from build123d import *

# Parameters (mm, degrees)
SKETCH1_R           = 4.5
BOSS_EXTRUDE3_DEPTH = 40
SKETCH4_R           = 3.5
CUT_EXTRUDE3_DEPTH  = 0.5
SKETCH5_R           = 3
CUT_EXTRUDE4_DEPTH  = 5
SKETCH6_R           = 2
BOSS_EXTRUDE4_DEPTH = 1
SKETCH7_R           = 0.6
BOSS_EXTRUDE5_DEPTH = 3.5
CHAMFER1_SIZE       = 0.4
CHAMFER1_SIZE2      = 0.145588094
FILLET1_R           = 0.2
CHAMFER2_SIZE       = 40
CHAMFER2_SIZE_2     = 0.698202597
FILLET2_R           = 0.5


# Read off the part's stored shape, not the designer's step: Dome1
with BuildPart() as part:
    # Sketch1 → Boss-Extrude3 (new body)
    with BuildSketch(Plane(origin=(0, 0, 0), x_dir=(1, 0, 0), z_dir=(0, 1, 0))):
        with Locations(Location((0, 0, 0), (0, 0, 270))):
            Circle(SKETCH1_R)
    extrude(amount=BOSS_EXTRUDE3_DEPTH)

    # Sketch4 → Cut-Extrude3 (cut)
    with BuildSketch(Plane.XZ):
        with Locations(Location((0, 0, 0), (0, 0, 270))):
            Circle(SKETCH4_R)
    extrude(amount=-CUT_EXTRUDE3_DEPTH, mode=Mode.SUBTRACT)

    # Sketch5 → Cut-Extrude4 (cut)
    with BuildSketch(Plane.XZ.offset(-0.5)):
        with Locations(Location((0, 0, 0), (0, 0, 270))):
            Circle(SKETCH5_R)
    extrude(amount=-CUT_EXTRUDE4_DEPTH, mode=Mode.SUBTRACT)

    # Sketch6 → Boss-Extrude4 (add)
    with BuildSketch(Plane.XZ.offset(-5.5)):
        with Locations(Location((0, 0, 0), (0, 0, 270))):
            Circle(SKETCH6_R)
    extrude(amount=BOSS_EXTRUDE4_DEPTH)

    # Sketch7 → Boss-Extrude5 (add)
    with BuildSketch(Plane.XZ.offset(-4.5)):
        with Locations(Location((0, 0, 0), (0, 0, 270))):
            Circle(SKETCH7_R)
    extrude(amount=BOSS_EXTRUDE5_DEPTH)

    # Chamfer1
    chamfer1_edges = [part.edges().sort_by_distance(p)[0] for p in [
        (0, 1, 0.6),
    ]]
    chamfer1_side = [part.faces().sort_by_distance(p)[0] for p in [
        (0, 2.75, 0.6),
    ]]
    chamfer(chamfer1_edges, length=CHAMFER1_SIZE, length2=CHAMFER1_SIZE2, reference=chamfer1_side[0])

    # Fillet1
    fillet1_edges = [part.edges().sort_by_distance(p)[0] for p in [
        (0, 1, 0.454411906),
    ]]
    fillet(fillet1_edges, radius=FILLET1_R)

    # Chamfer2
    # the kernel refuses this chamfer: 40, 0.698202597 mm, written as the material it takes off along each edge
    with BuildSketch(Plane(origin=(0, 40, 0), x_dir=(0, 0, 1), z_dir=(-1, 0, 0))) as chamfer2_piece_1:
        Polygon((4.5, -CHAMFER2_SIZE), (4.5 - CHAMFER2_SIZE_2, 0), (4.5, 0), align=None)
    revolve(axis=Axis((0, 40, 0), (0, 1, 0)), mode=Mode.SUBTRACT)

    # Dome1 outline → Dome1 (revolve)
    with BuildSketch(Plane.XY):
        with BuildLine():
            Line((0, 40), (3.801797408, 39.999999996))
            ThreePointArc((3.801797408, 39.999999996), (1.993342892, 40.892878392), (0, 41.2))
            Line((0, 41.2), (0, 40))
        make_face()
    revolve(axis=Axis((0, 0, 0), (0, 1, 0)))

    # Fillet2
    fillet2_edges = [part.edges().sort_by_distance(p)[0] for p in [
        (2.688276724, 40, 2.688276724),
    ]]
    fillet(fillet2_edges, radius=FILLET2_R)


solid = part.part
The listing builds one solid part. Answer for the finished solid, in the listing's coordinates (mm). Round coordinates to 2 decimals unless told otherwise and drop trailing zeros. Order: outer loops, then holes, each group sorted by start corner. A loop starts at its lowest first (then second) coordinate and runs counter-clockwise, first axis right, second up. Notation, with made-up numbers: M -28,49.25 L -15,49.25 A23 cw -15,87.25 Z; hole C -21,-18 d6. An arc over 180 degrees is marked long. Answer in a Markdown table with one row per item. Add a question column.
1) Determine the mould class of faces 1 (the face through (1.246, 20.148, 3.957)), 2 (the face through (-4, 0, 0)), 3 (the face through (-2, 5, 0)) for opening direction X: pulls with the +X half, pulls with the -X half, needs draft (parallel to the pull), parting line crosses it, or undercut.
2) Flat-ended cylindrical pins translate along their axes: pin 1 Ø1.5 at (x, y) = (-0.5, 11.5) entering from -Z; pin 2 Ø0.5 at (x, z) = (0, 0) entering from -Y; pin 3 Ø1 at (y, z) = (16.5, 1) entering from -X. Find the tip coordinate at first contact, or state that the pin passes through.
3) Consider line 1 along X through (y, z) = (0.25, 0); line 2 along X through (y, z) = (4.05, 0); line 3 along Z through (x, y) = (2.5, 8). Determine where each line is inside the solid, lowest interval first. Write a range as from..to.
4) The part is cut by section A-A on y = 25.5. Determine the outline of the cut face in (x, z).
5) The part is cut by section B-B on y = 36. Determine the outline of the cut face in (x, z), plus the area to 3 significant figures.
Findings below:
| question | item | result |
|---|---|---|
| 1 | face 1 | parting line crosses it |
| 1 | face 2 | needs draft |
| 1 | face 3 | undercut |
| 2 | pin 1 | stops at z = -4.31 |
| 2 | pin 2 | stops at y = 1 |
| 2 | pin 3 | stops at x = -4.18 |
| 3 | line 1 | x = -4.5..-3.5, 3.5..4.5 |
| 3 | line 2 | x = -4.43..-3, -0.6..0.6, 3..4.43 |
| 3 | line 3 | z = -3.57..3.57 |
| 4 | outline | C 0,0 d8.11 |
| 5 | outline | C 0,0 d7.74 |
| 5 | area | 47.1 mm² |
